Here's how the part is built. I have some questions about the finished solid (model axes, mm). Round coordinates to 2 decimals unless told otherwise and drop trailing zeros. Loops run counter-clockwise (first coordinate to the right, second up) from the corner with the lowest first, then second, coordinate; pieces in that order, holes last. Notation, with made-up numbers: M 47.5,67.25 L 82.5,67.25 A33 cw 82.5,100.25 Z; hole C 46.5,-34.75 d9. An arc over 180 degrees is marked long. Use a Markdown table: item, result.
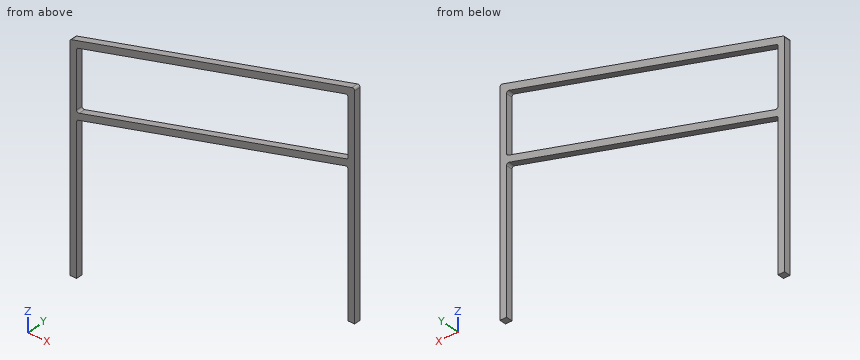
```python
from build123d import *

# Parameters (mm, degrees)
F1_DEPTH = 16


with BuildPart() as f1:
    # F0 (on Front) → F1 (new body, symmetric)
    with BuildSketch(Plane.XZ):
        with BuildLine():
            Line((-255.046532, 319.867053), (-255.046532, -742.5))
            Line((-255.046532, -742.5), (-222.546532, -742.5))
            Line((-222.546532, -742.5), (-222.546532, -31.247201))
            ThreePointArc((-222.546532, -31.247201), (-220.495519, -25.17978), (-215.183813, -21.60123))
            Line((-215.183813, -21.60123), (1093.658919, 336.246306))
            ThreePointArc((1093.658919, 336.246306), (1102.363621, 334.549323), (1106.2962, 326.600335))
            Line((1106.2962, 326.600335), (1106.2962, -361.412819))
            Line((1106.2962, -361.412819), (1138.7962, -361.412819))
            Line((1138.7962, -361.412819), (1138.7962, 695.486082))
            ThreePointArc((1138.7962, 695.486082), (1134.863621, 703.43507), (1126.158919, 705.132052))
            Line((1126.158919, 705.132052), (-247.683813, 329.513023))
            ThreePointArc((-247.683813, 329.513023), (-252.995519, 325.934473), (-255.046532, 319.867053))
        make_face()
        with BuildLine():
            ThreePointArc((1093.658919, 662.55348), (1102.363621, 660.856497), (1106.2962, 652.90751))
            Line((1106.2962, 652.90751), (1106.2962, 379.834382))
            ThreePointArc((1106.2962, 379.834382), (1104.245188, 373.766961), (1098.933482, 370.188411))
            Line((1098.933482, 370.188411), (-209.90925, 12.340875))
            ThreePointArc((-209.90925, 12.340875), (-218.613952, 14.037858), (-222.546532, 21.986846))
            Line((-222.546532, 21.986846), (-222.546532, 295.059974))
            ThreePointArc((-222.546532, 295.059974), (-220.495519, 301.127394), (-215.183813, 304.705944))
            Line((-215.183813, 304.705944), (1093.658919, 662.55348))
        make_face(mode=Mode.SUBTRACT)
    extrude(amount=F1_DEPTH, both=True)


solid = f1.part
```
Q1. Imagine slicing it at B-B, the plane y = 8. Please give me the cut outline in (x, z).
Return value:
| item | result |
|---|---|
| outline | M -255.05,-742.5 L -222.55,-742.5 L -222.55,-31.25 A10 cw -215.18,-21.6 L 1093.66,336.25 A10 cw 1106.3,326.6 L 1106.3,-361.41 L 1138.8,-361.41 L 1138.8,695.49 A10 ccw 1126.16,705.13 L -247.68,329.51 A10 ccw -255.05,319.87 Z; hole M -222.55,21.99 A10 ccw -209.91,12.34 L 1098.93,370.19 A10 ccw 1106.3,379.83 L 1106.3,652.91 A10 ccw 1093.66,662.55 L -215.18,304.71 A10 ccw -222.55,295.06 Z |
Q2. Imagine slicing it at A-A, the plane z = -117.5. Please give me the cut outline in (x, y).
Return value:
| item | result |
|---|---|
| outline | M -255.05,-16 L -222.55,-16 L -222.55,16 L -255.05,16 Z; M 1106.3,-16 L 1138.8,-16 L 1138.8,16 L 1106.3,16 Z |
Q3. Imagine slicing it at D-D, the plane z = 122.5. Please give me the cut outline in (x, y), then the cut area to 3 significant figures.
Return value:
| item | result |
|---|---|
| outline | M -255.05,-16 L -222.55,-16 L -222.55,16 L -255.05,16 Z; M 193,-16 L 311.87,-16 L 311.87,16 L 193,16 Z; M 1106.3,-16 L 1138.8,-16 L 1138.8,16 L 1106.3,16 Z |
| area | 5,880 mm^2 |
Q4. Will these pins go through, and if not, where does the flat tip stop? P1, Ø12, axis at x = 446, y = 6, coming from the -Z side; P2, Ø5, axis at x = 558.5, y = 11, coming from the +Z side; P3, Ø5, axis at x = 577, y = 1.5, coming from the +Z side.
Return value:
| item | result |
|---|---|
| P1 | stops at z = 157.53 |
| P2 | stops at z = 550.61 |
| P3 | stops at z = 555.67 |
Q5. Imagine slicing it at C-C, the plane x = 1010.5. Please give me the cut outline in (y, z).
Return value:
| item | result |
|---|---|
| outline | M -16,313.51 L 16,313.51 L 16,346.01 L -16,346.01 Z; M -16,639.82 L 16,639.82 L 16,673.51 L -16,673.51 Z |
Q6. I need wall thicknesses on line 1 (X direction, y = 3.5, z = -343.5); line 2 (X direction, y = -10.5, z = -603.5); line 3 (Z direction, x = 734.5, y = 5.5). Which ranges of each line are inside material? Lowest first, please. Write a range as from..to.
Return value:
| item | result |
|---|---|
| line 1 | x = -255.05..-222.55, 1106.3..1138.8 |
| line 2 | x = -255.05..-222.55 |
| line 3 | z = 238.05..270.55, 564.36..598.05 |
